Autodesk Inventor part; units mm, degrees
ref_plane "YZ Plane" through (0, 0, 0) normal (1, 0, 0) x (0, 1, 0)
ref_plane "XZ Plane" through (0, 0, 0) normal (0, 1, 0) x (-1, 0, 0)
ref_plane "XY Plane" through (0, 0, 0) normal (0, 0, 1) x (1, 0, 0)
sketch "Sketch1" plane through (0, 0, 0) normal (1, 0, 0) x (0, 1, 0)
  line L0 (-6, -12.5) -> (-6, -12.9)
  arc A0 (-6, -12.9) -> (-5.6, -13.3) centre (-5.6, -12.9) ccw
  line L1 (-5.6, -13.3) -> (-4.9, -13.3)
  arc A1 (-4.9, -13.3) -> (-4.7, -13.1) centre (-4.9, -13.1) ccw
  line L2 (-4.7, -13.1) -> (-4.7, -12.85)
  arc A2 (-4.5, -12.65) -> (-4.7, -12.85) centre (-4.5, -12.85) ccw
  line L3 (-4.5, -12.65) -> (-1.8, -12.65)
  arc A3 (-1.4, -13.05) -> (-1.8, -12.65) centre (-1.8, -13.05) ccw
  line L4 (-1.4, -13.05) -> (-1.4, -18.75)
  line L5 (-1.8, -19.15) -> (-4.5, -19.15)
  arc A4 (-1.8, -19.15) -> (-1.4, -18.75) centre (-1.8, -18.75) ccw
  arc A5 (-4.7, -18.95) -> (-4.5, -19.15) centre (-4.5, -18.95) ccw
  line L6 (-4.7, -18.95) -> (-4.7, -18.7)
  arc A6 (-4.7, -18.7) -> (-4.9, -18.5) centre (-4.9, -18.7) ccw
  line L7 (-4.9, -18.5) -> (-5.6, -18.5)
  arc A7 (-5.6, -18.5) -> (-6, -18.9) centre (-5.6, -18.9) ccw
  line L8 (-6, -18.9) -> (-6, -19.5)
  line L9 (-6.5, -6.5) -> (-6.5, -12.5)
  line L10 (-6.5, -12.5) -> (-2.5, -12.5)
  line L11 (-1.05, -19.5) -> (-6.5, -19.5)
  line L12 (-6.5, -19.5) -> (-6.5, -26)
  line L13 (-6.5, -26) -> (-1.05, -26)
  line L14 (-6, -26) -> (-6, -26.6)
  arc A8 (-6, -26.6) -> (-5.6, -27) centre (-5.6, -26.6) ccw
  line L15 (-5.6, -27) -> (-4.9, -27)
  arc A9 (-4.9, -27) -> (-4.7, -26.8) centre (-4.9, -26.8) ccw
  arc A10 (-4.5, -26.35) -> (-4.7, -26.55) centre (-4.5, -26.55) ccw
  line L16 (-4.7, -26.8) -> (-4.7, -26.55)
  line L17 (-4.5, -26.35) -> (-1.8, -26.35)
  arc A11 (-1.4, -26.75) -> (-1.8, -26.35) centre (-1.8, -26.75) ccw
  line L18 (-1.4, -26.75) -> (-1.4, -32.45)
  arc A12 (-1.8, -32.85) -> (-1.4, -32.45) centre (-1.8, -32.45) ccw
  line L19 (-1.8, -32.85) -> (-4.5, -32.85)
  arc A13 (-4.7, -32.65) -> (-4.5, -32.85) centre (-4.5, -32.65) ccw
  line L20 (-4.7, -32.65) -> (-4.7, -32.4)
  arc A14 (-4.7, -32.4) -> (-4.9, -32.2) centre (-4.9, -32.4) ccw
  line L21 (-4.9, -32.2) -> (-5.6, -32.2)
  arc A15 (-5.6, -32.2) -> (-6, -32.6) centre (-5.6, -32.6) ccw
  line L22 (-6, -32.6) -> (-6, -33)
  line L23 (-2.5, -33) -> (-6.5, -33)
  line L24 (-6.5, -33) -> (-6.5, -39)
  line L25 (32.5, 0) -> (0, 0)
  circle A16 centre (0, -6.5) radius 4.75
  circle A17 centre (32.5, -6.5) radius 4.75
  circle A18 centre (0, -39) radius 4.75
  circle A19 centre (32.5, -39) radius 4.75
  line L26 (39, -26) -> (39, -19.5)
  line L27 (39, -12.5) -> (39, -6.5)
  line L28 (39, -39) -> (39, -33)
  line L29 (26.5, -45.5) -> (32.5, -45.5)
  line L30 (0, -45.5) -> (6, -45.5)
  line L31 (13, -45.5) -> (19.5, -45.5)
  circle A20 centre (16.2588, 5.0016) radius 2.5
  circle A21 centre (16.25, -50.5) radius 2.5
  line L32 (44, 10) -> (-11.5, 10)
  line L33 (-11.5, 10) -> (-11.5, -55.5)
  line L34 (-11.5, -55.5) -> (44, -55.5)
  line L35 (44, -55.5) -> (44, 10)
  line L36 (44, 10) -> (-11.5, 10)
  line L37 (-11.5, 10) -> (-11.5, 30)
  line L38 (-11.5, 30) -> (44, 30)
  line L39 (44, 30) -> (44, 10)
  line L40 (44, -55.5) -> (-11.5, -55.5)
  line L41 (-11.5, -55.5) -> (-11.5, -75.5)
  line L42 (-11.5, -75.5) -> (44, -75.5)
  line L43 (44, -75.5) -> (44, -55.5)
  circle A22 centre (16.25, 20) radius 5
  circle A23 centre (16.25, -65.5) radius 5
  point P0 (24.75, -17.8425)
  point P1 (-11.5, 10)
  dimension "d0" = 20
  dimension "d1" = 20
  dimension "d2" = 10
  dimension "d3" = 10
extrude "Extrusion1" add sketch "Sketch1" along normal blind 10 contours A16 | A17 | A18 | A19 | L35 L34 L33 L32 | L32 L37 L38 L39 | L43 L42 L41 L34
properties part number "PlacaBaseHidráulicos_CPY"
Verification items for the finished model (mm, model axes). Give positions to 0.01 mm unless a question says otherwise; leave off trailing zeros. Loops run counter-clockwise (first coordinate to the right, second up) from the corner with the lowest first, then second, coordinate; pieces in that order, holes last.
1. Thickness scan on line 1 (Z direction, x = 7.5, y = 16.25); line 2 (Y direction, x = 5, z = 19); line 3 (Y direction, x = 0.5, z = -63). Record the ranges inside material, lowest first.
2. Mould release check, pull along Y, two halves, no side actions. Record for faces 1 (the flat face through (5, -11.5, -22)), 2 (the cylindrical face through (4.93, 18.938, -69.716)), 3 (the flat face through (5, 16, 30)): released by +Y, released by -Y, zero draft, split by the parting line, or undercut.
3. Section check C-C, the plane z = -65.5. Enter the section's corners in (x, y), then the cut area to 3 significant figures.
4. Section check B-B, the plane x = 1.25. Enter the section's corners in (y, z).
5. Section check A-A, the plane z = -50.5. Enter the section's corners in (x, y).
Geometry says:
1. line 1: z = -75.5 to -70.5, -60.5 to -53, -48 to 2.5, 7.5 to 15, 25 to 30
1. line 2: y = -11.5 to 11.35, 21.15 to 44
1. line 3: y = -11.5 to 11.92, 20.58 to 44
2. face 1: released by -Y
2. face 2: undercut
2. face 3: zero draft
3. outline: (0, -11.5) - (10, -11.5) - (10, 11.25) - (0, 11.25) - close; (0, 21.25) - (10, 21.25) - (10, 44) - (0, 44) - close
3. area: 455 mm2
4. outline: (-11.5, -75.5) - (44, -75.5) - (44, 30) - (-11.5, 30) - close; hole circle Ø10 at (16.25, -65.5); hole circle Ø10 at (16.25, 20); hole circle Ø5 at (16.25, -50.5); hole circle Ø5 at (16.26, 5)
5. outline: (0, -11.5) - (10, -11.5) - (10, 13.75) - (0, 13.75) - close; (0, 18.75) - (10, 18.75) - (10, 44) - (0, 44) - close
